Verification items for the finished model (mm, model axes). Face numbers are marked on the shaded views. Coordinates: 2 decimals unless noted, no trailing zeros. Loops run counter-clockwise (first coordinate to the right, second up) from the corner with the lowest first, then second, coordinate; pieces in that order, holes last. Notation, with made-up numbers: M 53.25,62.25 L 60.25,62.25 A24 cw 60.25,89.25 Z; hole C 15.25,-32.5 d9. An arc over 180 degrees is marked long. Write item = value, one per line. Start each with the question number.
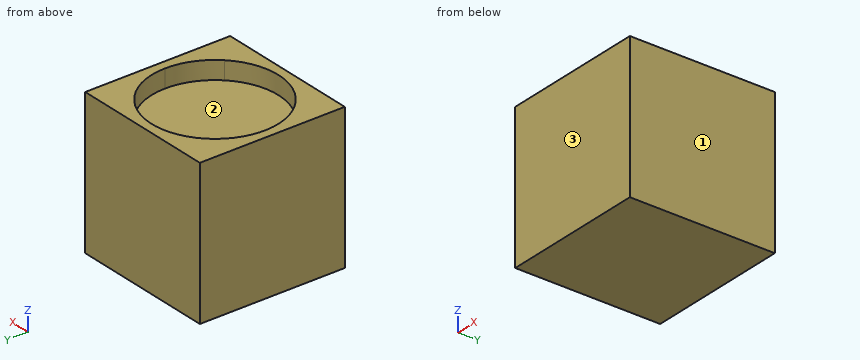
```python
from build123d import *

# Parameters (mm, degrees)
F0_W     = 50.8
F0_H     = 50.8
F1_DEPTH = 50.8
F3_DEPTH = 6.35


with BuildPart() as f1:
    # F0 (on Top) → F1 (new body)
    with BuildSketch(Plane.XY):
        with Locations((-25.4, -25.4)):
            Rectangle(F0_W, F0_H)
    extrude(amount=F1_DEPTH)

    # F2 (on face) → F3 (cut)
    with BuildSketch(Plane.XY.offset(50.8)):
        with BuildLine():
            ThreePointArc((-9.684552, -41.115448), (-4.866777, -33.905139), (-3.175, -25.4))
            ThreePointArc((-3.175, -25.4), (-16.894861, -4.866777), (-41.115448, -9.684552))
            Line((-41.115448, -9.684552), (-9.684552, -41.115448))
        make_face()
        with BuildLine():
            Line((-9.684552, -41.115448), (-41.115448, -9.684552))
            ThreePointArc((-41.115448, -9.684552), (-41.115448, -41.115448), (-9.684552, -41.115448))
        make_face()
    extrude(amount=-F3_DEPTH, mode=Mode.SUBTRACT)


solid = f1.part
```
Q1. Sectioned sample at B-B on y = -28.5. Record the cut outline in (x, z).
Q2. Scan lines: L1, parallel to X at y = -25, z = 46; L2, parallel to Z at x = -5.5, y = -35; L3, parallel to X at y = -31.5, z = 48.5. Record each from-to range of solid material in increasing order. Write a range as [from, to].
Q3. Mould release check, pull along Y, two halves, no side actions. Record for the marked faces 1, 2 and 3: +Y half, -Y half, draft (parallel to the pull), parting line (faces both ways), or undercut.
Q4. Gauge pin test, flat end, axial feed: pin 1 (22 mm diameter, centred on x = -22.5, y = -31.5, fed in from +Z). Record the tip position at first contact, or that the pin passes through.
Q5. Sectioned sample at A-A on x = -25.4. Record the cut outline in (y, z) (3 decimals), plus the area to 3 significant figures.
Solutions:
q1.outline = M -50.8,0 L 0,0 L 0,50.8 L -3.39,50.8 L -3.39,44.45 L -47.41,44.45 L -47.41,50.8 L -50.8,50.8 Z
q2.L1 = [-50.8, -47.62], [-3.18, 0]
q2.L2 = [0, 44.45]
q2.L3 = [-50.8, -46.77], [-4.03, 0]
q3.face_1 = draft
q3.face_2 = undercut
q3.face_3 = -Y half
q4.pin_1 = 44.45
q5.outline = M -50.8,0 L 0,0 L 0,50.8 L -3.175,50.8 L -3.175,44.45 L -47.625,44.45 L -47.625,50.8 L -50.8,50.8 Z
q5.area = 2,300 mm²
